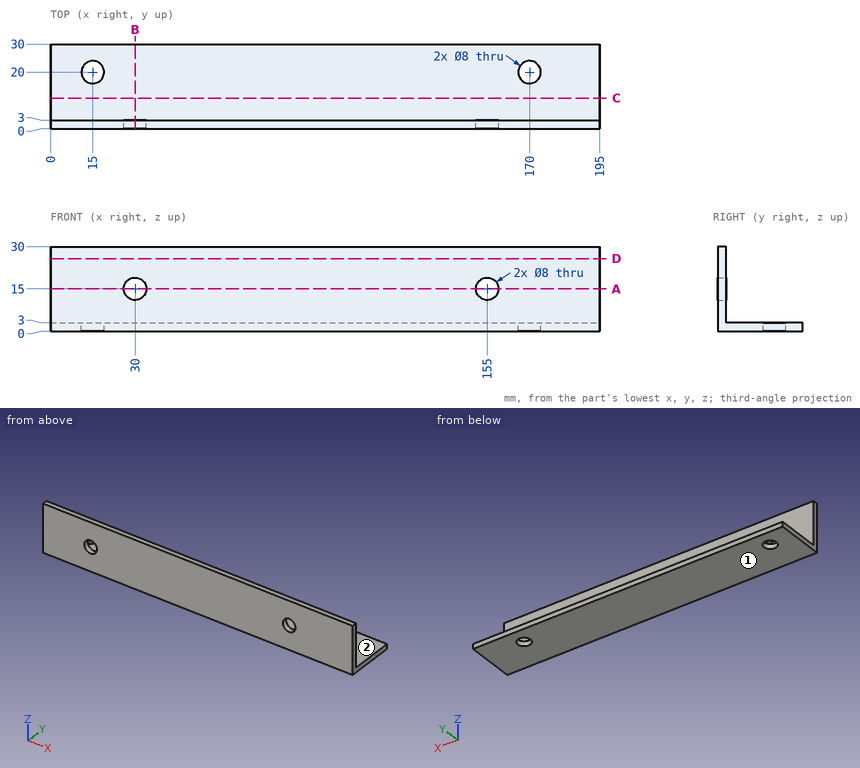
Answer from the drawing. Dimensions are ordinates in mm from the lowest x, y and z of the part. A direction names the side the tool comes from. Coordinates: 2 decimals unless noted, no trailing zeros. Order: outer loops, then holes, each group sorted by start corner. A loop starts at its lowest first (then second) coordinate and runs counter-clockwise, first axis right, second up. Notation, with made-up numbers: (22, -17) - (64, -17) arc R13 ccw to (64, -1) - close; hole circle Ø11 at (-13, 30.25). An arc over 180 degrees is marked (long way). Put each result on its own line as item: value. Start each with the question number.
1) For the marked faces 1 and 2, determine the directions among +Z, -Z, +X, -X, +Y, -Y from which every point of the face is accessible in a straight line to the end or side of a thin tool.
2) Find section A-A (z = 15). Give the vertices of the cut face in (x, y), plus the area to 3 significant figures.
3) Find section C-C (y = 10.75). Give the vertices of the cut face in (x, z).
4) Find the intervals of material crossed by line 1 (X direction, y = 20, z = 2.25); line 2 (X direction, y = 22, z = 1.75); line 3 (Z direction, x = 155, y = 2.1), in increasing order. Write a range as from..to.
5) Flat-ended cylindrical pins translate along their axes: pin 1 (8 mm diameter, centred on y = 7.5, z = 7.5, fed in from -X); pin 2 (8 mm diameter, centred on x = 69, y = 18, fed in from +Z); pin 3 (8 mm diameter, centred on x = 132, z = 15.5, fed in from +Y). Find the tip coordinate at first contact, or state that the pin passes through.
6) Find section B-B (x = 30). Give the vertices of the cut face in (y, z).
Results list:
1. face 1: -Z, +X, -X, +Y, -Y
1. face 2: +Z, +X, -X, +Y
2. outline: (0, 0) - (26, 0) - (26, 3) - (0, 3) - close; (34, 0) - (151, 0) - (151, 3) - (34, 3) - close; (159, 0) - (195, 0) - (195, 3) - (159, 3) - close
2. area: 537 mm^2
3. outline: (0, 0) - (195, 0) - (195, 3) - (0, 3) - close
4. line 1: x = 0..11, 19..166, 174..195
4. line 2: x = 0..11.54, 18.46..166.54, 173.46..195
4. line 3: z = 0..11, 19..30
5. pin 1: passes through
5. pin 2: stops at z = 3
5. pin 3: stops at y = 3
6. outline: (0, 0) - (30, 0) - (30, 3) - (3, 3) - (3, 11) - (0, 11) - close; (0, 19) - (3, 19) - (3, 30) - (0, 30) - close
